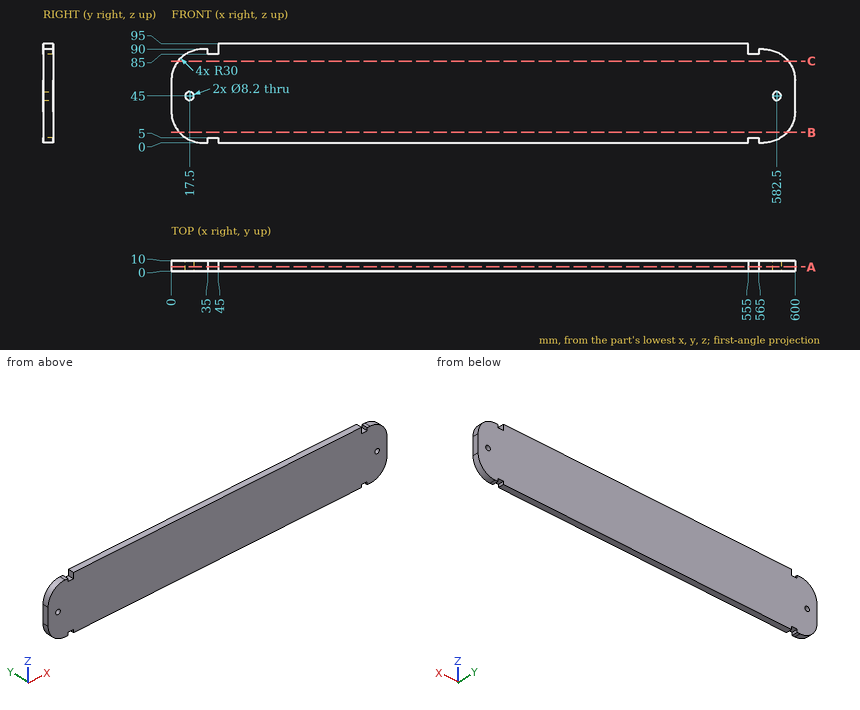
Job drawing, mm, ordinate dimensions from the low corner. One solid piece. Round coordinates to 2 decimals unless told otherwise and drop trailing zeros. Order: outer loops, then holes, each group sorted by start corner. A loop starts at its lowest first (then second) coordinate and runs counter-clockwise, first axis right, second up. Notation, with made-up numbers: (-20.5, -6) -> (-6.5, -6) arc R29 cw to (-6.5, 19) -> close; hole circle Ø10 at (45, 48.5). An arc over 180 degrees is marked (long way). Write item = value, one per line.
(1) Drill centre lines: L1, parallel to Z at x = 43.5, y = 1; L2, parallel to X at y = 4, z = 87.5; L3, parallel to Z at x = 17.5, y = 5. Where is each one in solid material? Low to high.
Answers follow:
L1 = 5 to 85
L2 = 18.01 to 35, 45 to 555, 565 to 581.99
L3 = 2.73 to 40.9, 49.1 to 87.27
(2) Cut at C-C (z = 78.5). Write the cut outline in (x, y).
Answers follow:
outline = (6.38, 0) -> (593.62, 0) -> (593.62, 10) -> (6.38, 10) -> close
(3) Cut at A-A (y = 4). Write the cut outline in (x, z).
Answers follow:
outline = (0, 30) arc R30 ccw to (30, 0) -> (35, 0) -> (35, 5) -> (45, 5) -> (45, 0) -> (555, 0) -> (555, 5) -> (565, 5) -> (565, 0) -> (570, 0) arc R30 ccw to (600, 30) -> (600, 60) arc R30 ccw to (570, 90) -> (565, 90) -> (565, 85) -> (555, 85) -> (555, 95) -> (45, 95) -> (45, 85) -> (35, 85) -> (35, 90) -> (30, 90) arc R30 ccw to (0, 60) -> close; hole circle Ø8.2 at (17.5, 45); hole circle Ø8.2 at (582.5, 45)
(4) Cut at B-B (z = 10). Write the cut outline in (x, y).
Answers follow:
outline = (7.64, 0) -> (592.36, 0) -> (592.36, 10) -> (7.64, 10) -> close
(5) Flat gauge pins, fed straight in: P1, Ø2.5, axis at x = 32.5, y = 3, coming from the +Z side; P2, Ø5.5, axis at y = 6.5, z = 87, coming from the -X side; P3, Ø1.5, axis at y = 6, z = 88, coming from the +X side; P4, Ø6.5, axis at x = 17.5, z = 45, coming from the +Y side. Where does each tip first touch, or does it go through?
Answers follow:
P1 = 90
P2 = 12.34
P3 = 582.55
P4 = through
